Autodesk Inventor part; units mm, degrees
ref_plane "YZ Plane" through (0, 0, 0) normal (1, 0, 0) x (0, 1, 0)
ref_plane "XZ Plane" through (0, 0, 0) normal (0, 1, 0) x (-1, 0, 0)
ref_plane "XY Plane" through (0, 0, 0) normal (0, 0, 1) x (1, 0, 0)
sketch "Sketch1" plane through (0, 0, 0) normal (0, 1, 0) x (-1, 0, 0)
  line L0 (6.35, 3.6662) -> (6.35, -3.6662)
  line L1 (6.35, -3.6662) -> (0, -7.3323)
  line L2 (0, -7.3323) -> (-6.35, -3.6662)
  line L3 (-6.35, -3.6662) -> (-6.35, 3.6662)
  line L4 (-6.35, 3.6662) -> (0, 7.3323)
  line L5 (0, 7.3323) -> (6.35, 3.6662)
  point P0 (0, 0)
  point P1 (0, 0)
  point P2 (-6.35, 0)
  dimension "d0" = 12.7
extrude "Extrusion1" add sketch "Sketch1" along normal blind 355.6
sketch "Sketch2" plane through (0, 355.6, 0) normal (0, 1, 0) x (1, 0, 0)
  circle A0 centre (0, 0) radius 2.5527
  dimension "d3" = 5.1054
extrude "Extrusion2" cut sketch "Sketch2" against normal blind 50.8
sketch "Sketch3" plane through (0, 0, 0) normal (0, -1, 0) x (1, 0, 0)
  circle A0 centre (0, 0) radius 2.5527
  circle A1 centre (0, 0) radius 2.5527
extrude "Extrusion3" cut sketch "Sketch3" against normal blind 50.8
thread "Thread1"
properties part number "CORL_014_Shaft" material "Aluminum 6061"
For this review, take the finished solid that the model builds, in its own axes (mm). Coordinates: 2 decimals unless noted, no trailing zeros. Write each loop counter-clockwise with the first axis right and the second up, starting at its lowest first coordinate (ties: lowest second). Pieces come first, ordered by that corner, then holes.
(1) Add section B-B on y = 98.5. Give the boundary of the cut face in (x, z), then the cut area to 3 significant figures.
(2) Wall thickness on probe 1 along Z at (x, y) = (0, 334.5); probe 2 along X at (y, z) = (326.5, 0); probe 3 along Z at (x, y) = (3, 259): over which ranges is each line inside the solid? List them lowest first.
(3) For pin 1 Ø1 at (x, y) = (-2.5, 286.5) entering from +Z; pin 2 Ø1.5 at (x, z) = (0.5, 0) entering from +Y; pin 3 Ø3 at (x, z) = (1.5, -2.5) entering from -Y; pin 4 Ø1.5 at (x, y) = (-4, 70) entering from -Z, all flat-tipped, find the tip position at first contact; note any pin that passes through.
(4) Add section A-A on z = 0. Give the boundary of the cut face in (x, y), then the cut area to 3 significant figures.
Answer sheet:
1. outline: (-6.35, -3.67) - (0, -7.33) - (6.35, -3.67) - (6.35, 3.67) - (0, 7.33) - (-6.35, 3.67) - close
1. area: 140 mm2
2. probe 1: z = -7.33 to -2.55, 2.55 to 7.33
2. probe 2: x = -6.35 to -2.55, 2.55 to 6.35
2. probe 3: z = -5.6 to 5.6
3. pin 1: stops at z = 6.18
3. pin 2: stops at y = 304.8
3. pin 3: stops at y = 0
3. pin 4: stops at z = -5.46
4. outline: (-6.35, 0) - (-2.55, 0) - (-2.55, 50.8) - (2.55, 50.8) - (2.55, 0) - (6.35, 0) - (6.35, 355.6) - (2.55, 355.6) - (2.55, 304.8) - (-2.55, 304.8) - (-2.55, 355.6) - (-6.35, 355.6) - close
4. area: 4,000 mm2
